Model file for the job. Use its own axes, mm. Face numbers are marked on the shaded views. A direction names the side the tool comes from. Coordinates: 2 decimals unless noted, no trailing zeros. Write each loop counter-clockwise with the first axis right and the second up, starting at its lowest first coordinate (ties: lowest second). Pieces come first, ordered by that corner, then holes. Notation, with made-up numbers: M -5.5,57 L 4.5,57 A17 cw 4.5,76 Z; hole C -23,14 d9. An arc over 180 degrees is marked long. Put each result on its own line as item: value. Start each with the question number.
Q1. Pull direction X, two halves, no side cores. Call the marked faces 3, 4 and 5: pulls with the +X half, pulls with the -X half, needs draft (parallel to the pull), parting line crosses it, or undercut.
Q2. Drill centre lines: line 1 along Z through (x, y) = (3.5, -3); line 2 along Y through (x, z) = (5.75, 0.25); line 3 along Y through (x, z) = (6, 4.5). Where is each one in solid material? Low to high.
Q3. Cut at A-A (x = 0). Write the cut outline in (y, z).
Q4. Which spindle directions (+Z, -Z, +X, -X, +Y, -Y) get a long thin tool onto all of the face, cutting with end or side? Do the marked faces 1 and 2. Say none if no direction does.
Q5. Drop flat-ended pins along their axis: pin 1 (3 mm diameter, centred on y = 0.5, z = -1.5, fed in from -X); pin 2 (1 mm diameter, centred on y = -3, z = -1, fed in from -X); pin 3 (2.5 mm diameter, centred on x = 1.5, y = 1, fed in from -Z). Give the stop position or say it passes through.
Q6. Cut at D-D (x = 2). Write the cut outline in (y, z), then the cut area to 3 significant figures.
Q7. Cut at B-B (z = -1.75). Write the cut outline in (x, y), then the cut area to 3 significant figures.
Q8. Cut at C-C (y = -2.5). Write the cut outline in (x, z).
```python
from build123d import *

# Parameters (mm, degrees)
SKETCH001_R  = 0.45
PAD001_DEPTH = 3.5
SKETCH_W     = 8
SKETCH_H     = 8
PAD_DEPTH    = 7.5
FILLET_R     = 0.9


with BuildPart() as pad001:
    # Sketch001 → Pad001 (new body)
    with BuildSketch(Plane.XY.offset(0.5)):
        Circle(SKETCH001_R)
        with Locations((5, 0)):
            Circle(SKETCH001_R)
    extrude(amount=-PAD001_DEPTH)


with BuildPart() as obj1:
    # Sketch → Pad (new body)
    with BuildSketch(Plane.XY.offset(0.1)):
        with Locations((2.5, 0)):
            Rectangle(SKETCH_W, SKETCH_H)
    extrude(amount=PAD_DEPTH)

    # Fillet
    fillet_edges = [obj1.edges().sort_by_distance(p)[0] for p in [
        (6.5, -4, 3.85),
        (6.5, 4, 3.85),
        (-1.5, -4, 3.85),
        (-1.5, 4, 3.85),
    ]]
    fillet(fillet_edges, radius=FILLET_R)

    # obj1: union Pad001
    add(pad001.part)


solid = obj1.part
```
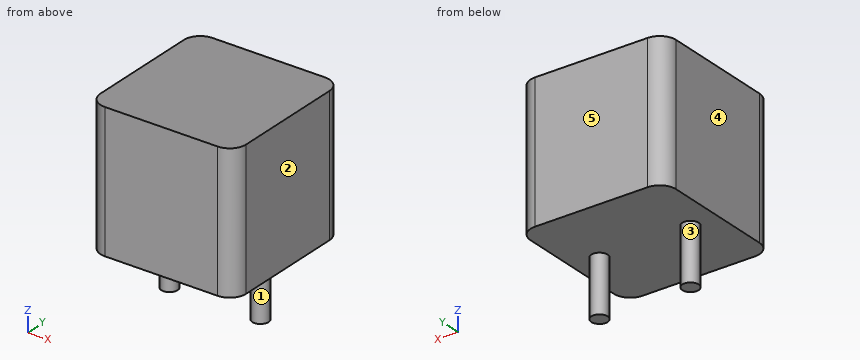
Computed values:
1. face 3: undercut
1. face 4: pulls with the -X half
1. face 5: needs draft
2. line 1: 0.1 to 7.6
2. line 2: -3.99 to 3.99
2. line 3: -3.91 to 3.91
3. outline: M -4,0.1 L -0.45,0.1 L -0.45,-3 L 0.45,-3 L 0.45,0.1 L 4,0.1 L 4,7.6 L -4,7.6 Z
4. face 1: -Z
4. face 2: +Z, -Z, +X, +Y, -Y
5. pin 1: x = -0.45
5. pin 2: through
5. pin 3: z = 0.1
6. outline: M -4,0.1 L 4,0.1 L 4,7.6 L -4,7.6 Z
6. area: 60.0 mm2
7. outline: C 0,0 d0.9; C 5,0 d0.9
7. area: 1.27 mm2
8. outline: M -1.5,0.1 L 6.5,0.1 L 6.5,7.6 L -1.5,7.6 Z
